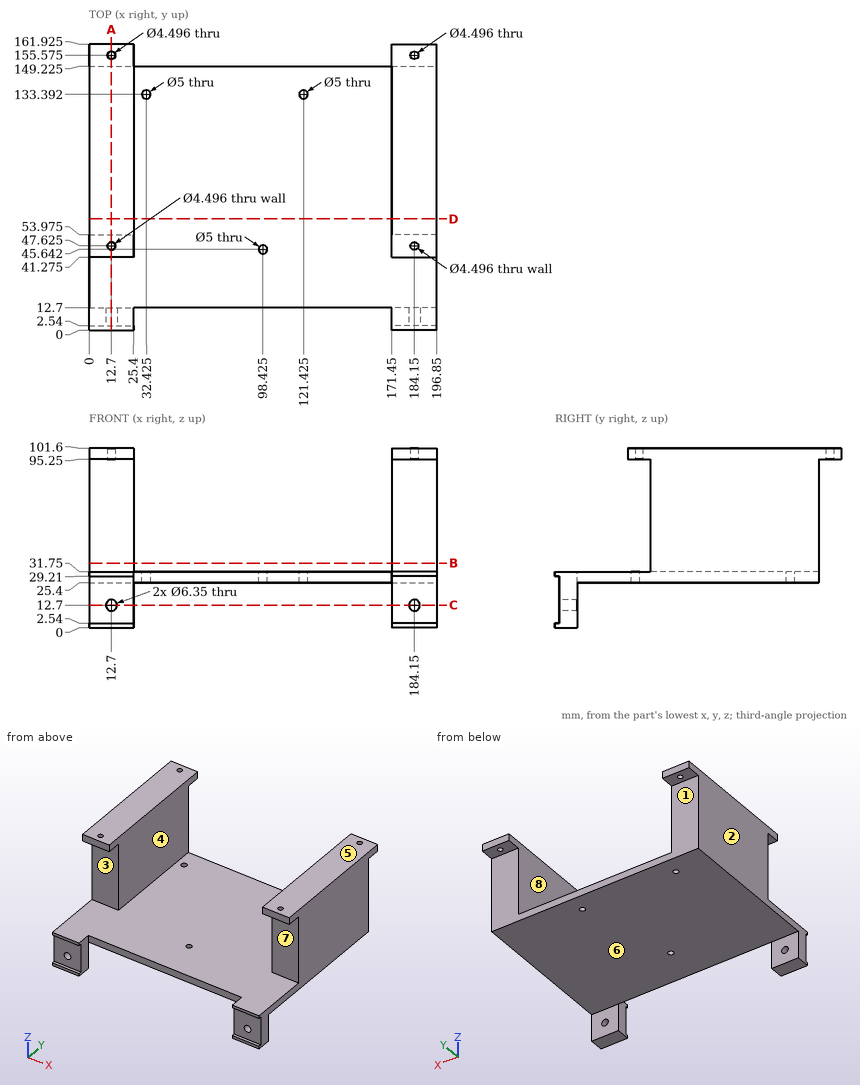
The figure shows three views and two pictorial views of one solid part (mm, origin at its lowest corner). Answer the questions. A direction names the side the tool comes from. Coordinates: 2 decimals unless noted, no trailing zeros. Order: outer loops, then holes, each group sorted by start corner. A loop starts at its lowest first (then second) coordinate and runs counter-clockwise, first axis right, second up.
Q1. A cutting plane is placed at A-A, the plane x = 12.7. State how many separate pieces and enclosed holes the cut face has, and give its area (3 significant figures).
Q2. Consider line 1 (X direction, y = 112.5, z = 60); line 2 (Z direction, x = 15.5, y = 47); line 3 (Z direction, x = 78, y = 97). Determine where each line is inside the solid, lowest interval first.
Q3. A cutting plane is placed at B-B, the plane z = 36.5. Write down the section's boundary in (x, y) (3 decimals), and give its area (3 significant figures).
Q4. Which of the six approach directions +Z, -Z, +X, -X, +Y, -Y give full straight-line access (tool end or side, diameter ignored) to the marked faces 1, 2, 3, 4 and 5?
Q5. For a pull along Z with two mould halves and no side action, classify the marked faces 6, 7 and 8 as pulls with the +Z half, pulls with the -Z half, needs draft (parallel to the pull), parting line crosses it, or undercut.
Q6. A cutting plane is placed at D-D, the plane y = 63. Write down the section's boundary in (x, z), and give its area (3 significant figures).
Q7. A cutting plane is placed at C-C, the plane z = 12.7. Write down the section's boundary in (x, y) (3 decimals), and give its area (3 significant figures).
Q8. Given P1, Ø1.9, axis at x = 179.5, z = 97.5, coming from the -Y side (3 decimals); P2, Ø7.5, axis at x = 185, z = 12.5, coming from the -Y side; P3, Ø10, axis at x = 180, y = 158.5, coming from the -Z side, each flat-ended and moving along its own axis, determine where each tip first touches the part or whether it passes through.
Answers follow:
1. separate pieces: 4
1. enclosed holes: 0
1. area: 7,900 mm2
2. line 1: x = 0 to 25.4, 171.45 to 196.85
2. line 2: z = 25.4 to 31.75, 95.25 to 101.6
2. line 3: z = 25.4 to 31.75
3. outline: (0, 53.975) - (25.4, 53.975) - (25.4, 149.225) - (0, 149.225) - close; (171.45, 53.975) - (196.85, 53.975) - (196.85, 149.225) - (171.45, 149.225) - close
3. area: 4,840 mm2
4. face 1: -Z, +X, -X, +Y
4. face 2: +Z, -Z, -X, +Y, -Y
4. face 3: +X, -X, -Y
4. face 4: +Z, +Y, -Y
4. face 5: +Z, +X, -X, +Y, -Y
5. face 6: pulls with the -Z half
5. face 7: undercut
5. face 8: needs draft
6. outline: (0, 25.4) - (196.85, 25.4) - (196.85, 101.6) - (171.45, 101.6) - (171.45, 31.75) - (25.4, 31.75) - (25.4, 101.6) - (0, 101.6) - close
6. area: 4,800 mm2
7. outline: (0, 2.54) - (9.525, 2.54) - (9.525, 12.7) - (0, 12.7) - close; (15.875, 2.54) - (25.4, 2.54) - (25.4, 12.7) - (15.875, 12.7) - close; (171.45, 2.54) - (180.975, 2.54) - (180.975, 12.7) - (171.45, 12.7) - close; (187.325, 2.54) - (196.85, 2.54) - (196.85, 12.7) - (187.325, 12.7) - close
7. area: 387 mm2
8. P1: stops at y = 41.275
8. P2: stops at y = 2.54
8. P3: stops at z = 95.25
